Design review of the part built by this model. Coordinates are the model's own, in mm. A direction names the side the tool comes from. Round coordinates to 2 decimals unless told otherwise and drop trailing zeros. Order: outer loops, then holes, each group sorted by start corner. A loop starts at its lowest first (then second) coordinate and runs counter-clockwise, first axis right, second up. Notation, with made-up numbers: M 88,-7.75 L 115,-7.75 A23 ccw 115,26.25 Z; hole C 89.5,-27 d5. An arc over 180 degrees is marked long. Write item = value, one per line. Start each with the question number.
```python
from build123d import *

# Parameters (mm, degrees)
SKIZZE1_R               = 2.5
LINEAR_AUSTRAGEN1_DEPTH = 4


with BuildPart() as part:
    # Skizze1 → Linear austragen1 (new body)
    with BuildSketch(Plane.XY):
        with BuildLine():
            Line((-1.720471048, -5), (1.279528952, -5))
            ThreePointArc((1.279528952, -5), (5.067353874, -3.263798762), (6.224608269, 0.739047056))
            Line((6.224608269, 0.739047056), (3.328540718, 20.117087516))
            ThreePointArc((3.328540718, 20.117087516), (3.300790208, 24.356992637), (4.460596804, 28.435278329))
            Line((4.460596804, 28.435278329), (9.633958573, 40.054839106))
            ThreePointArc((9.633958573, 40.054839106), (9.969901697, 41.962682181), (9.36998022, 43.804642334))
            Line((9.36998022, 43.804642334), (1.695101739, 56.061428328))
            ThreePointArc((1.695101739, 56.061428328), (-0.886899712, 56.792598366), (-1.872184322, 54.296490325))
            Line((-1.872184322, 54.296490325), (1.85912682, 44.36670191))
            ThreePointArc((1.85912682, 44.36670191), (1.800761722, 40.701037253), (-0.742535185, 38.060555344))
            Line((-0.742535185, 38.060555344), (-3.938539061, 36.599525001))
            ThreePointArc((-3.938539061, 36.599525001), (-5.909088644, 36.774512117), (-6.765186682, 38.5579869))
            Line((-6.765186682, 38.5579869), (-6.617488885, 40.670163795))
            ThreePointArc((-6.617488885, 40.670163795), (-6.711017842, 40.853724709), (-6.917001695, 40.85732017))
            Line((-6.917001695, 40.85732017), (-10.133974596, 39))
            ThreePointArc((-10.133974596, 39), (-10.599900423, 38.392793641), (-10.5, 37.633974596))
            Line((-10.5, 37.633974596), (-7.085329154, 31.719591199))
            ThreePointArc((-7.085329154, 31.719591199), (-5.460159239, 27.593857014), (-5.112249457, 23.173244093))
            Line((-5.112249457, 23.173244093), (-6.708291299, 0.348782369))
            ThreePointArc((-6.708291299, 0.348782369), (-5.377239556, -3.4099918), (-1.720471048, -5))
        make_face()
        Circle(SKIZZE1_R, mode=Mode.SUBTRACT)
    extrude(amount=LINEAR_AUSTRAGEN1_DEPTH)


solid = part.part
```
(1) Draft analysis for pull direction Y (two halves, no side actions). For faces 5 (the face through (0, 26, 0)), 6 (the face through (5.586, 49.847, 1.972)), 7 (the face through (-0.033, 49.401, 1.972)), state which applies: pulls with the +Y half, pulls with the -Y half, needs draft (parallel to the pull), parting line crosses it, or undercut.
(2) Insertion check: pin 1 (3 mm diameter, centred on x = -1.5, y = 27.5, fed in from -Z); pin 2 (2 mm diameter, centred on y = 50, z = 3, fed in from +X). Each pin has a flat end and moves straight along its axis. Give the tip position at first contact, or say it passes through.
(3) Consider section C-C, the plane x = -9.5. Write out the cut boundary in (y, z).
(4) Consider section B-B, the plane z = 1.45. Write out the cut boundary in (x, y).
(5) For faces 1 (the face through (7.01, 34.16, 1.97)), 2 (the face through (-5.89, 36.76, 1.97)), 3 (the face through (-5.9, 11.9, 2)), 4 (the face through (-8.817, 34.718, 1.972)), list the 3-axis set-ups (+Z, -Z, +X, -X, +Y, -Y) from which the entire face can be reached by the end or side of a thin tool; tool diameter is ignored.
(6) Consider section A-A, the plane x = 0. Write out the cut boundary in (y, z).
(7) Consider section D-D, the plane y = 13. Write out the cut boundary in (x, z), then the cut area to 3 significant figures.
(8) For line 1 along Y through (x, z) = (2.25, 0.9); line 2 along X through (y, z) = (43, 3); line 3 along Y through (x, z) = (9.25, 1.95), list the stretches that pass through material, from the lowest coordinate up. Write a range as [from, to].
Completed:
q1.face_5 = needs draft
q1.face_6 = pulls with the +Y half
q1.face_7 = undercut
q2.pin_1 = 0
q2.pin_2 = 6.12
q3.outline = M 35.9,0 L 39.37,0 L 39.37,4 L 35.9,4 Z
q4.outline = M -10.5,37.63 L -7.09,31.72 A15 cw -5.11,23.17 L -6.71,0.35 A5 ccw -1.72,-5 L 1.28,-5 A5 ccw 6.22,0.74 L 3.33,20.12 A15 cw 4.46,28.44 L 9.63,40.05 A4 ccw 9.37,43.8 L 1.7,56.06 A2 ccw -1.87,54.3 L 1.86,44.37 A5 cw -0.74,38.06 L -3.94,36.6 A2 cw -6.77,38.56 L -6.62,40.67 A0.2 ccw -6.92,40.86 L -10.13,39 A1 ccw Z; hole C 0,0 d5
q5.face_1 = +Z, -Z, +X
q5.face_2 = +Z, -Z
q5.face_3 = +Z, -Z, -X
q5.face_4 = +Z, -Z, -X, -Y
q6.outline = M -5,0 L -2.5,0 L -2.5,4 L -5,4 Z; M 2.5,0 L 38.48,0 L 38.48,4 L 2.5,4 Z; M 49.31,0 L 57,0 L 57,4 L 49.31,4 Z
q7.outline = M -5.82,0 L 4.39,0 L 4.39,4 L -5.82,4 Z
q7.area = 40.9 mm2
q8.line_1 = [-4.9, -1.09], [1.09, 55.18]
q8.line_2 = [2.16, 9.76]
q8.line_3 = [39.19, 44]
